For this review, use the dimensioned drawing (mm, ordinates from the lowest corner) and the shaded views. A direction names the side the tool comes from. Give positions to 0.01 mm unless a question says otherwise; leave off trailing zeros. Write each loop counter-clockwise with the first axis right and the second up, starting at its lowest first coordinate (ties: lowest second). Pieces come first, ordered by that corner, then holes.
1) We need section C-C on y = 12.25. Give the boundary of the cut face in (x, z).
2) For P1, Ø4, axis at x = 20, z = 12.5, coming from the -Y side, flat-tipped, find the tip position at first contact; note if it passes through.
3) We need section B-B on z = 10. Give the boundary of the cut face in (x, y).
4) We need section A-A on y = 8.5. Give the boundary of the cut face in (x, z), and give its area (3 significant figures).
5) Draft analysis for pull direction Z (two halves, no side actions). For the marked faces 1, 2 and 3, state which applies: pulls with the +Z half, pulls with the -Z half, needs draft (parallel to the pull), parting line crosses it, or undercut.
6) Machinability: for the marked faces 4, 5 and 6, which of the approach directions +Z, -Z, +X, -X, +Y, -Y give a long, thin tool a straight path to every point of the face, cutting with its end or side? Answer none if there is none.
7) Wall thickness on line 1 along X through (y, z) = (7.5, 5); line 2 along Z through (x, y) = (2.5, 8.25); line 3 along X through (y, z) = (9.25, 9.5): over which ranges is each line inside the solid? List them lowest first.
8) We need section D-D on z = 1.75. Give the boundary of the cut face in (x, y).
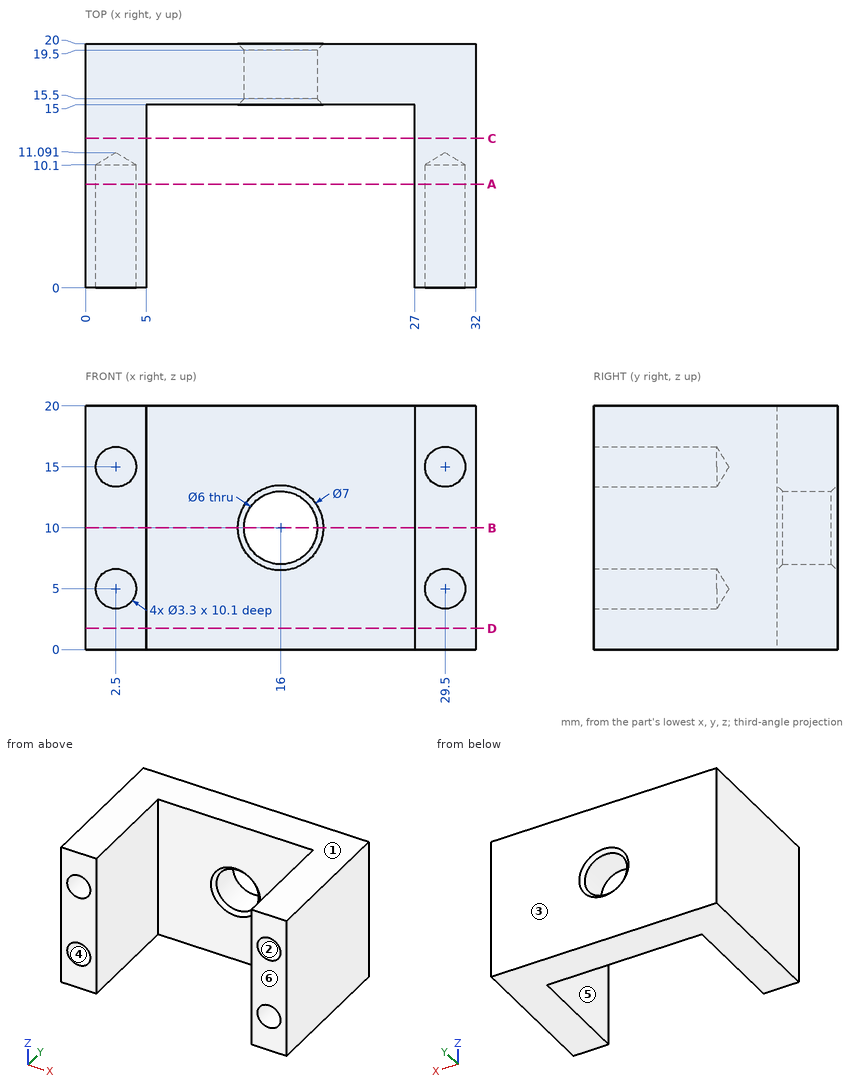
Results list:
1. outline: (0, 0) - (5, 0) - (5, 20) - (0, 20) - close; (27, 0) - (32, 0) - (32, 20) - (27, 20) - close
2. P1: stops at y = 15
3. outline: (0, 0) - (5, 0) - (5, 15) - (12.5, 15) - (13, 15.5) - (13, 19.5) - (12.5, 20) - (0, 20) - close; (19, 15.5) - (19.5, 15) - (27, 15) - (27, 0) - (32, 0) - (32, 20) - (19.5, 20) - (19, 19.5) - close
4. outline: (0, 0) - (5, 0) - (5, 20) - (0, 20) - close; (27, 0) - (32, 0) - (32, 20) - (27, 20) - close; hole circle Ø3.3 at (2.5, 5); hole circle Ø3.3 at (2.5, 15); hole circle Ø3.3 at (29.5, 5); hole circle Ø3.3 at (29.5, 15)
4. area: 166 mm2
5. face 1: pulls with the +Z half
5. face 2: undercut
5. face 3: needs draft
6. face 4: -Y
6. face 5: +Z, -Z, -Y
6. face 6: +Z, -Z, +X, -X, -Y
7. line 1: x = 0 to 0.85, 4.15 to 5, 27 to 27.85, 31.15 to 32
7. line 2: z = 0 to 3.35, 6.65 to 13.35, 16.65 to 20
7. line 3: x = 0 to 5, 27 to 32
8. outline: (0, 0) - (5, 0) - (5, 15) - (27, 15) - (27, 0) - (32, 0) - (32, 20) - (0, 20) - close
